Autodesk Inventor part; units mm, degrees
ref_plane "XZ Plane" through (0, 0, 0) normal (0, 1, 0) x (-1, 0, 0)
sketch "Sketch1" plane through (0, 0, 0) normal (0, 1, 0) x (-1, 0, 0)
  circle A0 centre (0, 0) radius 12.5
  dimension "d0" = 25
extrude "Extrusion1" add sketch "Sketch1" along normal blind 55
sketch "Sketch2" plane through (0, 55, 0) normal (0, 1, 0) x (1, 0, 0)
  circle A0 centre (0, 0) radius 12.5
  circle A1 centre (0, 0) radius 4
  dimension "d3" = 8
extrude "Extrusion2" add sketch "Sketch2" along normal blind 3 contours A1
sketch "Sketch3" plane through (0, 58, 0) normal (0, 1, 0) x (1, 0, 0)
  circle A0 centre (0, 0) radius 4
  circle A1 centre (0, 0) radius 2
  line L0 (-2, 0) -> (0.25, 1.9843)
  line L1 (-17.5, 0) -> (17.5, 0)
  dimension "d6" = 4
  dimension "d7" = 3
extrude "Extrusion3" add sketch "Sketch3" along normal blind 8 contours L1 L0 A1 | A1 L1
sketch "Sketch4" plane through (0, 55, 0) normal (0, 1, 0) x (1, 0, 0)
  circle A0 centre (0, 0) radius 4
  circle A1 centre (0, 0) radius 12.5
  circle A2 centre (0, 0) radius 8.5 construction
  line L0 (-17.5, 0) -> (17.5, 0) construction
  line L1 (0, 17.5) -> (0, -17.5) construction
  point P0 (0, -8.5)
  point P1 (0, 8.5)
  dimension "d10" = 17
hole "Hole1" at (0, 55, -8.5) at (0, 55, 8.5) direction (0, -1, 0) diameter 3 depth 8 tip angle 118
properties part number "motor_small" material "Iron, Malleable"
Here's how the part is built. I have some questions about the finished solid (model axes, mm). A direction names the side the tool comes from. Round coordinates to 2 decimals unless told otherwise and drop trailing zeros. Order: outer loops, then holes, each group sorted by start corner. A loop starts at its lowest first (then second) coordinate and runs counter-clockwise, first axis right, second up. Notation, with made-up numbers: M 83.5,6.25 L 103.5,6.25 A14 ccw 103.5,32.25 Z; hole C -31,63 d8. An arc over 180 degrees is marked long. One line per question, with ' | ' between items.
1) I want a section at C-C, the plane x = 6. Write out the boundary of the cut face in (y, z), then the cut area to 3 significant figures.
Working result:
outline: M 0,-10.97 L 55,-10.97 L 55,10.97 L 0,10.97 Z | area: 1,210 mm²
2) For pin 1 Ø4 at (x, y) = (7.5, 40) entering from +Z (3 decimals); pin 2 Ø5 at (x, y) = (2, 10) entering from +Z; pin 3 Ø4 at (y, z) = (58, -8) entering from +X; pin 4 Ø4 at (x, y) = (2.5, 55) entering from -Z, each with a flat end and sliding along its axis, tell me the tip position at first contact or that it passes through.
Working result:
pin 1: z = 11.225 | pin 2: z = 12.5 | pin 3: through | pin 4: z = -12.49
3) For faces 1 (the face through (0, 66, 0)), 2 (the face through (3, 55, 3)), which set-ups out of +Z, -Z, +X, -X, +Y, -Y let a thin tool reach every point of the face, with its end or its side?
Working result:
face 1: +Z, -Z, +X, -X, +Y | face 2: +Y
4) I want a section at B-B, the plane y = 14. Write out the boundary of the cut face in (x, z).
Working result:
outline: C 0,0 d25
5) If we mould it in two halves opening along X, with no side actions, what happens to faces 3 (the face through (1.37, 61.944, 1.457)), 4 (the face through (-0.89, 61.94, -0.98)), 5 (the face through (0.22, 46.255, 8.64))? For each: +X half, -X half, draft (parallel to the pull), parting line (faces both ways), or undercut.
Working result:
face 3: parting line | face 4: -X half | face 5: undercut
6) I want a section at D-D, the plane x = -7. Write out the boundary of the cut face in (y, z).
Working result:
outline: M 0,-10.36 L 55,-10.36 L 55,10.36 L 0,10.36 Z
7) I need wall thicknesses on line 1 along Z through (x, y) = (0, 53); line 2 along Y through (x, z) = (2.75, -1.75); line 3 along Y through (x, z) = (4.75, 2). Which ranges of each line are inside material? Lowest first, please.
Working result:
line 1: -12.5 to -10, -7 to 7, 10 to 12.5 | line 2: 0 to 58 | line 3: 0 to 55
8) I want a section at A-A, the plane y = 51.5. Write out the boundary of the cut face in (x, z), then the cut area to 3 significant figures.
Working result:
outline: C 0,0 d25; hole C 0,-8.5 d3; hole C 0,8.5 d3 | area: 477 mm²
